Autodesk Inventor part; units mm, degrees
ref_plane "YZ Plane" through (0, 0, 0) normal (1, 0, 0) x (0, 1, 0)
ref_plane "XZ Plane" through (0, 0, 0) normal (0, 1, 0) x (-1, 0, 0)
ref_plane "XY Plane" through (0, 0, 0) normal (0, 0, 1) x (1, 0, 0)
sketch "Sketch1" plane through (0, 0, 0) normal (0, 0, 1) x (1, 0, 0)
  line L0 (-12.7, -12.7) -> (12.7, -12.7)
  line L1 (12.7, 12.7) -> (-12.7, 12.7)
  line L2 (-12.7, 12.7) -> (-12.7, -12.7)
  line L3 (-12.7, -12.7) -> (12.7, 12.7) construction
  line L4 (12.7, -12.7) -> (-12.7, 12.7) construction
  line L5 (12.7, 12.7) -> (12.7, 16.51)
  line L6 (12.7, 16.51) -> (-16.51, 16.51)
  line L7 (-16.51, 16.51) -> (-16.51, 12.7)
  line L8 (12.7, -12.7) -> (12.7, -16.51)
  line L9 (12.7, -16.51) -> (-16.51, -16.51)
  line L10 (-16.51, -16.51) -> (-16.51, 12.7)
  point P0 (0, 0)
  dimension "d0" = 25.4
  dimension "d1" = 25.4
  dimension "d2" = 3.81
  dimension "d3" = 29.21
  dimension "d4" = 3.81
  dimension "d5" = 29.21
extrude "Extrusion1" add sketch "Sketch1" along normal blind 29.21
sketch "Sketch2" plane through (0, 0, 29.21) normal (0, 0, 1) x (1, 0, 0)
  line L0 (12.7, 12.7) -> (12.7, 16.51)
  line L1 (12.7, 16.51) -> (-16.51, 16.51)
  line L2 (-16.51, 16.51) -> (-16.51, -16.51)
  line L3 (-16.51, -16.51) -> (12.7, -16.51)
  line L4 (12.7, -16.51) -> (12.7, -12.7)
  line L5 (12.7, 12.7) -> (12.7, -12.7)
  point P0 (0, 0)
extrude "Extrusion2" add sketch "Sketch2" against normal blind 3.81
sketch "Sketch3" plane through (0, 0, 0) normal (0, 0, -1) x (-1, 0, 0)
  line L0 (12.7, -12.7) -> (-12.7, -12.7)
  line L1 (-12.7, -12.7) -> (-12.7, -16.51)
  line L2 (-12.7, -16.51) -> (16.51, -16.51)
  line L3 (16.51, -16.51) -> (16.51, 16.51)
  line L4 (16.51, 16.51) -> (-12.7, 16.51)
  line L5 (-12.7, 16.51) -> (-12.7, 12.7)
  line L6 (-12.7, 12.7) -> (12.7, 12.7)
  line L7 (12.7, 12.7) -> (12.7, -12.7)
  point P0 (0, 0)
extrude "Extrusion3" add sketch "Sketch3" along normal blind 25.4
sketch "Sketch4" plane through (-16.51, 16.51, 29.21) normal (0, 1, 0) x (1, 0, 0)
  circle A0 centre (14.605, 40.9575) radius 3.175
  circle A1 centre (14.605, 13.6525) radius 3.175
  point P0 (16.51, 29.21)
  dimension "d12" = 6.35
  dimension "d13" = 6.35
extrude "Extrusion4" cut sketch "Sketch4" against normal blind 50.8
properties part number "west coast corner"
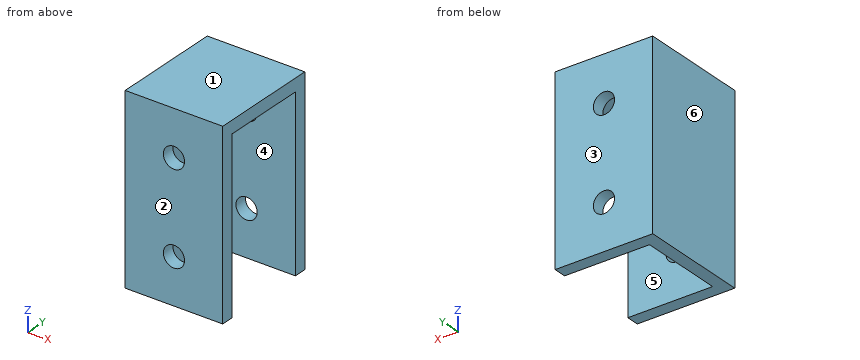
Could you check a few things on this model? Use its own coordinates, in mm. Face numbers are marked on the shaded views. A direction names the side the tool comes from. Give positions to 0.01 mm unless a question says otherwise; leave off trailing zeros. Loops run counter-clockwise (first coordinate to the right, second up) from the corner with the lowest first, then second, coordinate; pieces in that order, holes last. Notation, with made-up numbers: (13.5, 31.25) - (31.5, 31.25) arc R23 cw to (31.5, 40.25) - close; hole circle Ø11 at (18, 11). An arc over 180 degrees is marked (long way). Answer in a Markdown table with one row per item. Add a question column.
Q1. If we section it at A-A (z = -1): List the corners of the cut face in (x, y) for me.
Q2. If we section it at B-B (x = -4): List the corners of the cut face in (y, z) for me.
Q3. If we section it at D-D (y = -14): State how many separate pieces and enclosed holes the cut face has, plus the area to 3 significant figures.
Q4. For pin 1 (8.5 mm diameter, centred on x = -1.9, z = 15.56, fed in from +Y); pin 2 (2 mm diameter, centred on y = -9.5, z = 0, fed in from +X); pin 3 (7.5 mm diameter, centred on x = -1.5, y = -1.5, fed in from -Z), each with a flat end and sliding along its axis, tell me the tip position at first contact or that it passes through.
Q5. We'd pull the mould along Y, two halves only. Please class the marked faces 1, 2, 3 and 4: +Y half, -Y half, draft (parallel to the pull), parting line (faces both ways), or undercut.
Q6. If we section it at C-C (x = -7.75): List the corners of the cut face in (y, z) for me.
Q7. Which directions (+Z, -Z, +X, -X, +Y, -Y) give clear straight access to the entire face, cutting with the end or side of a thin tool? Please do the marked faces 5 and 6.
Q8. Please list where these lines run through material, in increasing order: L1, parallel to Y at x = -6, z = -22; L2, parallel to X at y = 12, z = 20; L3, parallel to Z at x = 3.5, y = 9. Write a range as from..to.
The answers:
| question | item | result |
|---|---|---|
| 1 | outline | (-16.51, -16.51) - (12.7, -16.51) - (12.7, -12.7) - (-12.7, -12.7) - (-12.7, 12.7) - (12.7, 12.7) - (12.7, 16.51) - (-16.51, 16.51) - close |
| 2 | outline | (-16.51, -25.4) - (-12.7, -25.4) - (-12.7, -14.13) - (-16.51, -14.13) - close; (-16.51, -9.36) - (-12.7, -9.36) - (-12.7, 13.17) - (-16.51, 13.17) - close; (-16.51, 17.94) - (-12.7, 17.94) - (-12.7, 25.4) - (12.7, 25.4) - (12.7, 17.94) - (16.51, 17.94) - (16.51, 29.21) - (-16.51, 29.21) - close; (12.7, -25.4) - (16.51, -25.4) - (16.51, -14.13) - (12.7, -14.13) - close; (12.7, -9.36) - (16.51, -9.36) - (16.51, 13.17) - (12.7, 13.17) - close |
| 3 | separate pieces | 1 |
| 3 | enclosed holes | 2 |
| 3 | area | 1,530 mm^2 |
| 4 | pin 1 | stops at y = 16.51 |
| 4 | pin 2 | stops at x = -12.7 |
| 4 | pin 3 | stops at z = 25.4 |
| 5 | face 1 | draft |
| 5 | face 2 | -Y half |
| 5 | face 3 | +Y half |
| 5 | face 4 | undercut |
| 6 | outline | (-16.51, -25.4) - (-12.7, -25.4) - (-12.7, 25.4) - (12.7, 25.4) - (12.7, -25.4) - (16.51, -25.4) - (16.51, 29.21) - (-16.51, 29.21) - close |
| 7 | face 5 | -Z, +X |
| 7 | face 6 | +Z, -Z, -X, +Y, -Y |
| 8 | L1 | y = -16.51..-12.7, 12.7..16.51 |
| 8 | L2 | x = -16.51..-12.7 |
| 8 | L3 | z = 25.4..29.21 |
